Design review of the part built by this model. Coordinates are the model's own, in mm. A direction names the side the tool comes from. Coordinates: 2 decimals unless noted, no trailing zeros. Loops run counter-clockwise (first coordinate to the right, second up) from the corner with the lowest first, then second, coordinate; pieces in that order, holes last. Notation, with made-up numbers: (-33.5, 66) - (-15.5, 66) arc R22 ccw to (-15.5, 78) - close; hole circle Ø4 at (51.5, 75). An arc over 180 degrees is marked (long way). Return JSON: item names as keys, results as strings. Group by question number.
from build123d import *

# Parameters (mm, degrees)
BOSS_EXTRUDE1_DEPTH    = 7.62
SKETCH2_W              = 12.7
SKETCH2_H              = 120.65
CUT_EXTRUDE1_DEPTH     = 0.254
SKETCH3_W              = 6.35
SKETCH3_H              = 120.65
CUT_EXTRUDE2_DEPTH     = 0.254
F_10_24_TAPPED_HOLE1_D = 3.7973


with BuildPart() as part:
    # Sketch1 → Boss-Extrude1 (new body)
    with BuildSketch(Plane(origin=(0, 0, 0), x_dir=(1, 0, 0), z_dir=(0, 1, 0))):
        Polygon((0, 60.325), (-9.525, 37.329615818), (-9.525, -37.329615818), (0, -60.325), (9.525, -37.329615818), (9.525, 37.329615818), align=None)
    extrude(amount=BOSS_EXTRUDE1_DEPTH)

    # Sketch2 → Cut-Extrude1 (cut)
    with BuildSketch(Plane.XZ):
        Rectangle(SKETCH2_W, SKETCH2_H)
    extrude(amount=-CUT_EXTRUDE1_DEPTH, mode=Mode.SUBTRACT)

    # Sketch3 → Cut-Extrude2 (cut)
    with BuildSketch(Plane.XZ.offset(-0.254)):
        Rectangle(SKETCH3_W, SKETCH3_H)
    extrude(amount=-CUT_EXTRUDE2_DEPTH, mode=Mode.SUBTRACT)

    # #10-24 Tapped Hole1 (through all)
    with Locations(Plane(origin=(0, 7.62, 0), x_dir=(1, 0, 0), z_dir=(0, 1, 0))):
        with Locations((0, 20.32), (0, 40.64), (0, 0), (0, -20.32), (0, -40.64)):
            Hole(F_10_24_TAPPED_HOLE1_D / 2)


solid = part.part
Item 1: To check wall thickness, follow line 1 (X direction, y = 6, z = -20.32) (3 decimals); line 2 (X direction, y = 5, z = -40.64); line 3 (Y direction, x = 3.25, z = -43). State the ranges of each line that lie inside material, in increasing order. Write a range as from..to.
Item 2: Add section D-D (x = 7.75). State the section outline as (y, z) points.
Item 3: Add section A-A (z = 20.32). State the section outline as (x, y) points (3 decimals).
Item 4: Draft analysis for pull direction X (two halves, no side actions). For faces 1 (the face through (-4.829, 3.757, 48.666)), 2 (the face through (5, 0.254, 1)), 3 (the face through (4.829, 3.757, -48.666)), state which applies: pulls with the +X half, pulls with the -X half, needs draft (parallel to the pull), parting line crosses it, or undercut.
Item 5: Add section C-C (z = -33). State the section outline as (x, y) points (3 decimals), then the cut area to 3 significant figures.
Item 6: For P1, Ø1, axis at x = 4, z = -13.5, coming from the -Y side; P2, Ø4.5, axis at x = 0, z = -40.64, coming from the -Y side; P3, Ø1, axis at x = 2.5, y = 1.5, coming from the -Z side, all flat-tipped, find the tip position at first contact; note any pin that passes through.
Item 7: Add section B-B (y = 6.25). State the section outline as (x, z) points (3 decimals).
Item 8: For faces 4 (the face through (-2, 0.508, 1)), 5 (the face through (-4.696, 3.757, -48.988)), list the 3-axis set-ups (+Z, -Z, +X, -X, +Y, -Y) from which the entire face can be reached by the end or side of a thin tool; tool diameter is ignored.
Answers below:
{
 "1": {"line 1": "x = -9.525..-1.899, 1.899..9.525", "line 2": "x = -8.15..-1.9, 1.9..8.15", "line 3": "y = 0.25..7.62"},
 "2": {"outline": "(0, -41.61) - (7.62, -41.61) - (7.62, 41.61) - (0, 41.61) - close"},
 "3": {"outline": "(-9.525, 0) - (-6.35, 0) - (-6.35, 0.254) - (-3.175, 0.254) - (-3.175, 0.508) - (-1.899, 0.508) - (-1.899, 7.62) - (-9.525, 7.62) - close; (1.899, 0.508) - (3.175, 0.508) - (3.175, 0.254) - (6.35, 0.254) - (6.35, 0) - (9.525, 0) - (9.525, 7.62) - (1.899, 7.62) - close"},
 "4": {"face 1": "pulls with the -X half", "face 2": "undercut", "face 3": "pulls with the +X half"},
 "5": {"outline": "(-9.525, 0) - (-6.35, 0) - (-6.35, 0.254) - (-3.175, 0.254) - (-3.175, 0.508) - (3.175, 0.508) - (3.175, 0.254) - (6.35, 0.254) - (6.35, 0) - (9.525, 0) - (9.525, 7.62) - (-9.525, 7.62) - close", "area": "140 mm^2"},
 "6": {"P1": "stops at y = 0.25", "P2": "stops at y = 0.51", "P3": "stops at z = -55.5"},
 "7": {"outline": "(-9.525, -37.33) - (0, -60.325) - (9.525, -37.33) - (9.525, 37.33) - (0, 60.325) - (-9.525, 37.33) - close; hole circle Ø3.797 at (0, -40.64); hole circle Ø3.797 at (0, -20.32); hole circle Ø3.797 at (0, 0); hole circle Ø3.797 at (0, 20.32); hole circle Ø3.797 at (0, 40.64)"},
 "8": {"face 4": "+Z, -Z, -Y", "face 5": "-Z, -X, +Y, -Y"}
}
